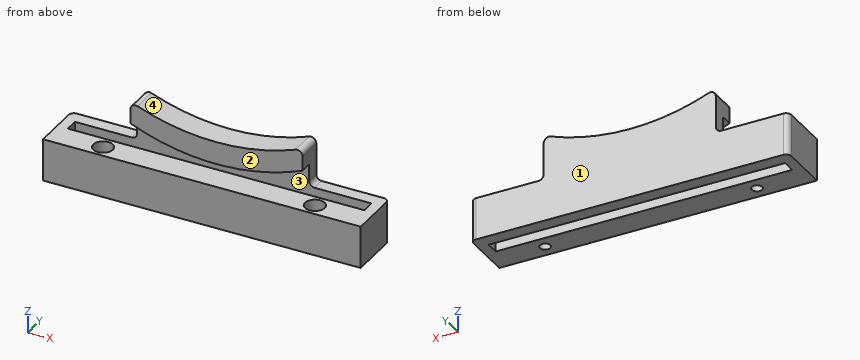
from build123d import *

# Parameters (mm, degrees)
SKETCH1_W           = 120
SKETCH1_H           = 20
SKETCH1_R           = 2
SKETCH1_W_2         = 112
SKETCH1_H_2         = 5
BOSS_EXTRUDE1_DEPTH = 16
SKETCH2_R           = 3.7
CUT_EXTRUDE1_DEPTH  = 8
BOSS_EXTRUDE2_DEPTH = 5
BOSS_EXTRUDE3_DEPTH = 4.7
FILLET1_R           = 2


with BuildPart() as part:
    # Sketch1 → Boss-Extrude1 (new body)
    with BuildSketch(Plane.XY):
        with Locations((0, 10)):
            Rectangle(SKETCH1_W, SKETCH1_H)
        with Locations((-40, 5)):
            Circle(SKETCH1_R, mode=Mode.SUBTRACT)
        with Locations((40, 5)):
            Circle(SKETCH1_R, mode=Mode.SUBTRACT)
        with Locations((0, 12.5)):
            Rectangle(SKETCH1_W_2, SKETCH1_H_2, mode=Mode.SUBTRACT)
    extrude(amount=BOSS_EXTRUDE1_DEPTH)

    # Sketch2 → Cut-Extrude1 (cut)
    with BuildSketch(Plane.XY.offset(16)):
        with Locations((-40, 5)):
            Circle(SKETCH2_R)
        with Locations((40, 5)):
            Circle(SKETCH2_R)
    extrude(amount=-CUT_EXTRUDE1_DEPTH, mode=Mode.SUBTRACT)

    # Sketch3 → Boss-Extrude2 (add)
    with BuildSketch(Plane(origin=(0, 20, 0), x_dir=(1, 0, 0), z_dir=(0, 1, 0))):
        with BuildLine():
            Line((-32.5, -33), (-32.5, -16))
            Line((-32.5, -16), (32.5, -16))
            Line((32.5, -16), (32.5, -33))
            ThreePointArc((32.5, -33), (0, -26.372442674), (-32.5, -33))
        make_face()
    extrude(amount=-BOSS_EXTRUDE2_DEPTH)

    # Sketch4 → Boss-Extrude3 (add)
    with BuildSketch(Plane.XZ.offset(-15)):
        with BuildLine():
            Line((-32.5, 24.52), (-32.5, 33))
            ThreePointArc((-32.5, 33), (0, 26.372442674), (32.5, 33))
            Line((32.5, 33), (32.5, 24.52))
            ThreePointArc((32.5, 24.52), (0, 17.892442674), (-32.5, 24.52))
        make_face()
    extrude(amount=BOSS_EXTRUDE3_DEPTH)

    # Fillet1
    fillet1_edges = [part.edges().sort_by_distance(p)[0] for p in [
        (32.5, 17.5, 16),
        (-32.5, 17.5, 16),
        (-32.5, 15.15, 33),
        (32.5, 15.15, 33),
        (-60, 20, 8),
        (60, 20, 8),
    ]]
    fillet(fillet1_edges, radius=FILLET1_R)


solid = part.part
Here's how the part is built. I have some questions about the finished solid (model axes, mm). Face numbers are marked on the shaded views. Give positions to 0.01 mm unless a question says otherwise; leave off trailing zeros. Loops run counter-clockwise (first coordinate to the right, second up) from the corner with the lowest first, then second, coordinate; pieces in that order, holes last. Notation, with made-up numbers: (-32.5, 49) -> (-5.5, 49) arc R27 cw to (-5.5, 68) -> close; hole circle Ø10 at (39.25, -5). An arc over 180 degrees is marked (long way). Answer as a JSON object with one key per item and string values. Group by question number.
Item 1: Thinking about a two-plate mould opening in Y: for the marked faces 1, 2, 3 and 4, which applies, pulls with the +Y half, pulls with the -Y half, needs draft (parallel to the pull), parting line crosses it, or undercut?
Item 2: Imagine slicing it at D-D on x = 16. Write out the boundary of the cut face in (y, z).
Item 3: Imagine slicing it at C-C on x = -40. Write out the boundary of the cut face in (y, z), then the cut area to 3 significant figures.
Item 4: Imagine slicing it at A-A on y = 5. Write out the boundary of the cut face in (x, z), then the cut area to 3 significant figures.
Item 5: I need wall thicknesses on L1, parallel to Y at x = 40, z = 10; L2, parallel to Y at x = -40, z = 1.5; L3, parallel to X at y = 5, z = 4.5. Which ranges of each line are inside material? Lowest first, please.
Item 6: Will these pins go through, and if not, where does the flat tip stop? pin 1 (1.5 mm diameter, centred on x = -32, y = 4.5, fed in from +Z); pin 2 (2 mm diameter, centred on x = 38.5, y = 3.5, fed in from +Z); pin 3 (10.5 mm diameter, centred on y = 14, z = 22.5, fed in from +X).
Item 7: Imagine slicing it at B-B on z = 6. Write out the boundary of the cut face in (x, y).
Answer list:
{
 "1": {"face 1": "pulls with the +Y half", "face 2": "pulls with the -Y half", "face 3": "undercut", "face 4": "needs draft"},
 "2": {"outline": "(0, 0) -> (10, 0) -> (10, 16) -> (0, 16) -> close; (10.3, 19.45) -> (15, 19.45) -> (15, 0) -> (20, 0) -> (20, 27.93) -> (10.3, 27.93) -> close"},
 "3": {"outline": "(0, 0) -> (3, 0) -> (3, 8) -> (1.3, 8) -> (1.3, 16) -> (0, 16) -> close; (7, 0) -> (10, 0) -> (10, 16) -> (8.7, 16) -> (8.7, 8) -> (7, 8) -> close; (15, 0) -> (20, 0) -> (20, 16) -> (15, 16) -> close", "area": "149 mm2"},
 "4": {"outline": "(-60, 0) -> (-42, 0) -> (-42, 8) -> (-43.7, 8) -> (-43.7, 16) -> (-60, 16) -> close; (-38, 0) -> (38, 0) -> (38, 8) -> (36.3, 8) -> (36.3, 16) -> (-36.3, 16) -> (-36.3, 8) -> (-38, 8) -> close; (42, 0) -> (60, 0) -> (60, 16) -> (43.7, 16) -> (43.7, 8) -> (42, 8) -> close", "area": "1,740 mm2"},
 "5": {"L1": "y = 0 to 1.3, 8.7 to 10, 15 to 20", "L2": "y = 0 to 3, 7 to 10, 15 to 20", "L3": "x = -60 to -42, -38 to 38, 42 to 60"},
 "6": {"pin 1": "stops at z = 16", "pin 2": "stops at z = 8", "pin 3": "stops at x = 32.61"},
 "7": {"outline": "(-60, 0) -> (60, 0) -> (60, 18) arc R2 ccw to (58, 20) -> (-58, 20) arc R2 ccw to (-60, 18) -> close; hole (-56, 10) -> (56, 10) -> (56, 15) -> (-56, 15) -> close; hole circle Ø4 at (-40, 5); hole circle Ø4 at (40, 5)"}
}
